Design review of the part shown in the three views and the two pictorial views. Dimensions are in mm from the part's minimum x, y and z. A direction names the side the tool comes from. Give positions to 0.01 mm unless a question says otherwise; leave off trailing zeros. Loops run counter-clockwise (first coordinate to the right, second up) from the corner with the lowest first, then second, coordinate; pieces in that order, holes last.
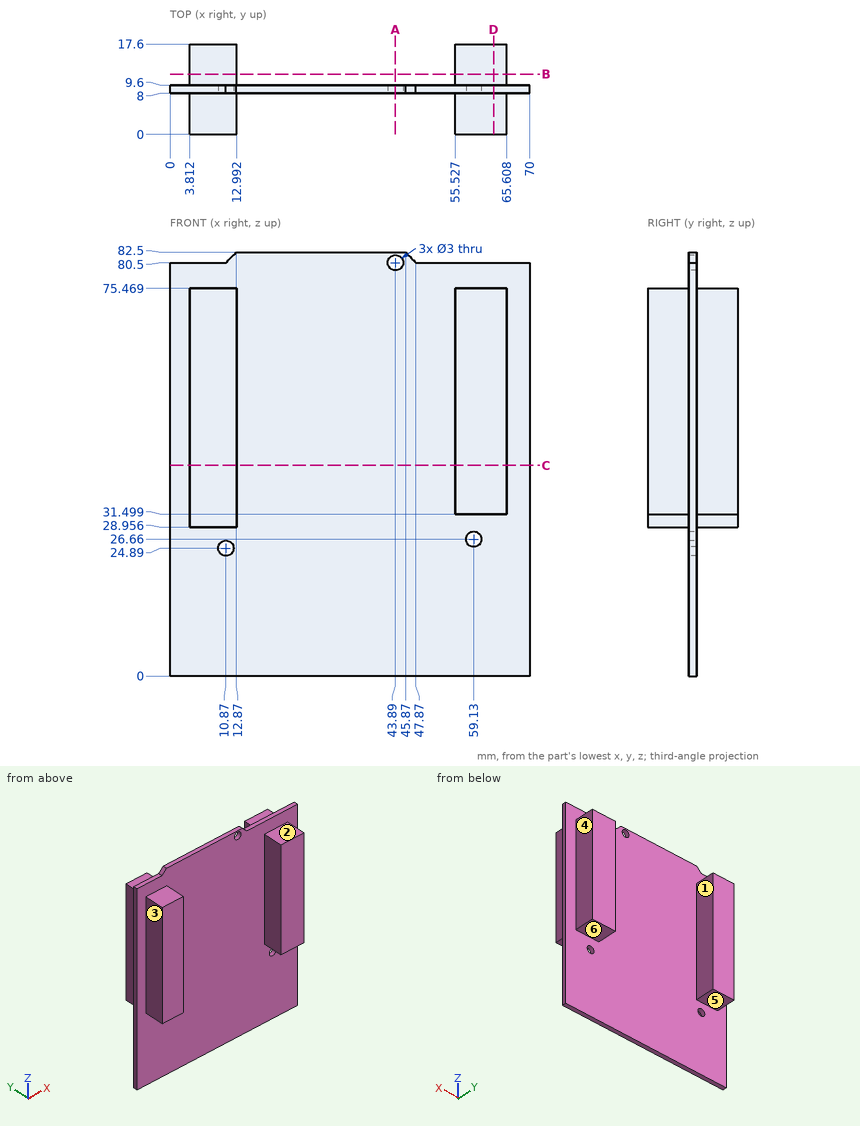
Q1. Take a section at D-D (x = 63). Give the boundary of the cut face in (y, z).
Results:
outline: (0, 31.5) - (8, 31.5) - (8, 0) - (9.6, 0) - (9.6, 31.5) - (17.6, 31.5) - (17.6, 75.47) - (9.6, 75.47) - (9.6, 80.5) - (8, 80.5) - (8, 75.47) - (0, 75.47) - close
Q2. Take a section at B-B (y = 11.75). Give the boundary of the cut face in (x, z), plus the area to 3 significant figures.
Results:
outline: (3.81, 28.96) - (12.99, 28.96) - (12.99, 75.47) - (3.81, 75.47) - close; (55.53, 31.5) - (65.61, 31.5) - (65.61, 75.47) - (55.53, 75.47) - close
area: 870 mm2
Q3. Take a section at A-A (x = 43.89). Give the boundary of the cut face in (y, z).
Results:
outline: (8, 0) - (9.6, 0) - (9.6, 79) - (8, 79) - close; (8, 82) - (9.6, 82) - (9.6, 82.5) - (8, 82.5) - close
Q4. Wall thickness on line 1 (X direction, y = 8.7, z = 24.89); line 2 (X direction, y = 9.2, z = 26.66); line 3 (Y direction, x = 50, z = 16.5): over which ranges is each line inside the solid? List them lowest first.
Results:
line 1: x = 0 to 9.37, 12.37 to 70
line 2: x = 0 to 57.63, 60.63 to 70
line 3: y = 8 to 9.6
Q5. Insertion check: pin 1 (6.5 mm diameter, centred on y = 2.5, z = 57.5, fed in from -X); pin 2 (9 mm diameter, centred on x = 9.5, y = 3, fed in from +Z); pin 3 (10 mm diameter, centred on x = 7.5, y = 6.5, fed in from -Z); pin 4 (4 mm diameter, centred on x = 59.13, z = 26.66, fed in from +Y). Each pin has a flat end and moves straight along its axis. Give the tip position at first contact, or say it passes through.
Results:
pin 1: stops at x = 3.81
pin 2: stops at z = 75.47
pin 3: stops at z = 0
pin 4: stops at y = 9.6
Q6. Draft analysis for pull direction X (two halves, no side actions). For the marked faces 1, 2 and 3, state which applies: pulls with the +X half, pulls with the -X half, needs draft (parallel to the pull), parting line crosses it, or undercut.
Results:
face 1: undercut
face 2: needs draft
face 3: pulls with the -X half
Q7. Take a section at C-C (z = 41). Give the boundary of the cut face in (x, y).
Results:
outline: (0, 8) - (3.81, 8) - (3.81, 0) - (12.99, 0) - (12.99, 8) - (55.53, 8) - (55.53, 0) - (65.61, 0) - (65.61, 8) - (70, 8) - (70, 9.6) - (65.61, 9.6) - (65.61, 17.6) - (55.53, 17.6) - (55.53, 9.6) - (12.99, 9.6) - (12.99, 17.6) - (3.81, 17.6) - (3.81, 9.6) - (0, 9.6) - close
Q8. Tool access review of the marked faces 4, 5 and 6: name each direction out of +Z, -Z, +X, -X, +Y, -Y from which nothing blocks a thin tool from reaching the whole face with its end or side.
Results:
face 4: +Z, -Z, +X, +Y
face 5: -Z, +X, -X, +Y
face 6: -Z, +X, +Y
